Build history of the part. All positions in model axes, mm. Face numbers are marked on the shaded views. Coordinates: 2 decimals unless noted, no trailing zeros. Order: outer loops, then holes, each group sorted by start corner. A loop starts at its lowest first (then second) coordinate and runs counter-clockwise, first axis right, second up. Notation, with made-up numbers: M 18.5,12 L 30.5,12 A6 cw 30.5,17 Z; hole C 33,-26 d9. An arc over 180 degrees is marked long. Write item = value, one per line. Start each with the question number.
Q1. Drill centre lines: probe 1 along X at (y, z) = (-9, 3); probe 2 along X at (y, z) = (-16, 5); probe 3 along Y at (x, z) = (91.5, 1.75). Where is each one in solid material? Low to high.
Q2. Band-saw the part on A-A on y = -1.5. Write the cut outline in (x, z).
Q3. Band-saw the part on B-B on x = 16. Write the cut outline in (y, z).
Q4. Pull direction X, two halves, no side cores. Call the marked faces 1, 2, 3 and 4: released by +X, released by -X, zero draft, split by the parting line, or undercut.
Q5. Band-saw the part on D-D on x = 50. Write the cut outline in (y, z).
Q6. Band-saw the part on C-C on z = 4.5. Write the cut outline in (x, y).
Q7. Pin check, flat tips, straight feed: P1, Ø1.5, axis at x = 79, y = 16.5, coming from the -Z side; P2, Ø1.9, axis at x = 73, z = 4.5, coming from the -Y side; P3, Ø3, axis at x = 17.5, z = 2.5, coming from the +Y side. Stop position of each tip, or through.
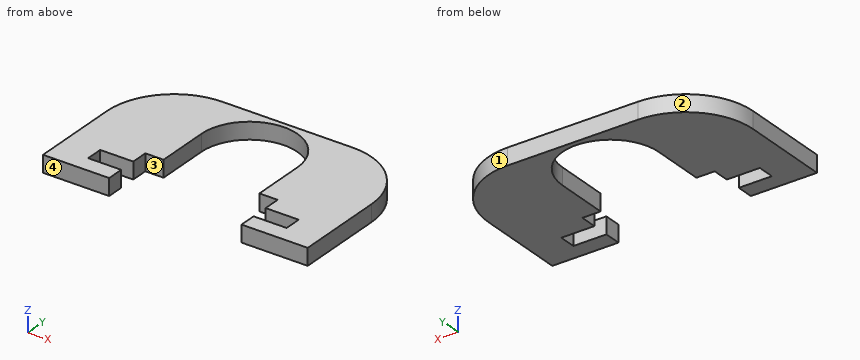
```python
from build123d import *

# Parameters (mm, degrees)
BOSS_EXTRUDE1_DEPTH     = 6.35
CUT_EXTRUDE1_DEPTH      = 108.890326167
CUT_EXTRUDE1_DEPTH_BACK = 108.890326167
FILLET1_R               = 25.4
CUT_EXTRUDE2_DEPTH      = 108.890326167
CUT_EXTRUDE2_DEPTH_BACK = 108.890326167
SKETCH4_W               = 12.499999987
SKETCH4_H               = 6.35


with BuildPart() as part:
    # Sketch1 → Boss-Extrude1 (new body)
    with BuildSketch(Plane.XY):
        Polygon((24.999999974, 0), (74.999999923, 0), (74.999999923, -6.35), (74.999999923, -19.05), (99.999999898, -19.05), (99.999999898, -6.35), (99.999999898, 0), (99.999999898, 40.00000001), (0, 40.00000001), (0, 0), (0, -6.35), (0, -19.05), (24.999999974, -19.05), (24.999999974, -6.35), align=None)
    extrude(amount=BOSS_EXTRUDE1_DEPTH)

    # Sketch2 → Cut-Extrude1 (cut, two sides: drawn at the far end of the back side and taken through both)
    with BuildSketch(Plane.XY.offset(6.35).offset(-CUT_EXTRUDE1_DEPTH_BACK)):
        with BuildLine():
            ThreePointArc((68.099999944, 20.000000005), (49.999999949, 38.1), (31.899999954, 20.000000005))
            Line((31.899999954, 20.000000005), (31.899999954, 0))
            Line((31.899999954, 0), (68.099999944, 0))
            Line((68.099999944, 0), (68.099999944, 20.000000005))
        make_face()
    extrude(amount=CUT_EXTRUDE1_DEPTH + CUT_EXTRUDE1_DEPTH_BACK, mode=Mode.SUBTRACT)

    # Fillet1
    fillet1_edges = [part.edges().sort_by_distance(p)[0] for p in [
        (0, 40.00000001, 3.175),
        (99.999999898, 40.00000001, 3.175),
    ]]
    fillet(fillet1_edges, radius=FILLET1_R)

    # Sketch4 → Cut-Extrude2 (cut, two sides: drawn at the far end of the back side and taken through both)
    with BuildSketch(Plane.XY.offset(6.35).offset(-CUT_EXTRUDE2_DEPTH_BACK)):
        with Locations((18.749999981, -9.525)):
            Rectangle(SKETCH4_W, SKETCH4_H)
        with Locations((81.249999918, -9.525)):
            Rectangle(SKETCH4_W, SKETCH4_H)
    extrude(amount=CUT_EXTRUDE2_DEPTH + CUT_EXTRUDE2_DEPTH_BACK, mode=Mode.SUBTRACT)


solid = part.part
```
Recorded:
q1.probe_1 = 0 to 12.5, 87.5 to 100
q1.probe_2 = 0 to 25, 75 to 100
q1.probe_3 = -19.05 to 33.56
q2.outline = M 0,0 L 25,0 L 25,6.35 L 0,6.35 Z; M 75,0 L 100,0 L 100,6.35 L 75,6.35 Z
q3.outline = M -19.05,0 L -12.7,0 L -12.7,6.35 L -19.05,6.35 Z; M -6.35,0 L 38.2,0 L 38.2,6.35 L -6.35,6.35 Z
q4.face_1 = released by +X
q4.face_2 = released by -X
q4.face_3 = undercut
q4.face_4 = zero draft
q5.outline = M 38.1,0 L 40,0 L 40,6.35 L 38.1,6.35 Z
q6.outline = M 0,-19.05 L 25,-19.05 L 25,-12.7 L 12.5,-12.7 L 12.5,-6.35 L 25,-6.35 L 25,0 L 31.9,0 L 31.9,20 A18.1 cw 68.1,20 L 68.1,0 L 75,0 L 75,-6.35 L 87.5,-6.35 L 87.5,-12.7 L 75,-12.7 L 75,-19.05 L 100,-19.05 L 100,14.6 A25.4 ccw 74.6,40 L 25.4,40 A25.4 ccw 0,14.6 Z
q7.P1 = 0
q7.P2 = 0
q7.P3 = 39.18
